Design review of the part built by this model. Coordinates are the model's own, in mm. A direction names the side the tool comes from. Coordinates: 2 decimals unless noted, no trailing zeros. Loops run counter-clockwise (first coordinate to the right, second up) from the corner with the lowest first, then second, coordinate; pieces in that order, holes last. Notation, with made-up numbers: M -11.75,-27 L 8.25,-27 A21 cw 8.25,-7 Z; hole C -22.75,57 d6. An arc over 180 degrees is marked long. Write item = value, one per line. Start each with the question number.
from build123d import *

# Parameters (mm, degrees)
SKETCH1_W                = 30
SKETCH1_H                = 80
BOSS_EXTRUDE1_DEPTH      = 5
SKETCH2_W                = 10
SKETCH2_H                = 10
BOSS_EXTRUDE2_DEPTH      = 30
CUT_EXTRUDE1_DEPTH       = 51.990195136
CUT_EXTRUDE1_DEPTH_BACK  = 51.990195136
SKETCH3_R                = 0.5
CUT_EXTRUDE2_DEPTH       = 46.276925691
CUT_EXTRUDE2_DEPTH_BACK  = 46.276925691
SKETCH4_W                = 25
SKETCH4_H                = 55
CUT_EXTRUDE3_DEPTH       = 83.006097334
CUT_EXTRUDE3_DEPTH_BACK  = 83.006097334
SKETCH5_W                = 26
SKETCH5_H                = 10
SKETCH6_W                = 10
SKETCH6_H                = 10
BOSS_EXTRUDE3_DEPTH      = 80
CUT_EXTRUDE4_DEPTH       = 83.006097334
CUT_EXTRUDE4_DEPTH_BACK  = 83.006097334
SKETCH7_R                = 1
CUT_EXTRUDE5_DEPTH       = 46.82575695
CUT_EXTRUDE5_DEPTH_BACK  = 46.82575695
SKETCH8_W                = 56
SKETCH8_H                = 10
SKETCH9_W                = 10
SKETCH9_H                = 10
CUT_EXTRUDE6_DEPTH       = 10
SKETCH10_W               = 10
SKETCH10_H               = 10
CUT_EXTRUDE7_DEPTH       = 10
SKETCH12_W               = 10
SKETCH12_H               = 2
BOSS_EXTRUDE5_DEPTH      = 10
CUT_EXTRUDE8_DEPTH       = 73.665328734
CUT_EXTRUDE8_DEPTH_BACK  = 73.665328734
SKETCH13_R               = 1
CUT_EXTRUDE11_DEPTH      = 46.276925691
CUT_EXTRUDE11_DEPTH_BACK = 46.276925691
SKETCH15_W               = 2
SKETCH15_H               = 2
SKETCH16_W               = 10
SKETCH16_H               = 10
BOSS_EXTRUDE6_DEPTH      = 30
SKETCH17_W               = 10
SKETCH17_H               = 10
CUT_EXTRUDE12_DEPTH      = 28
CUT_EXTRUDE13_DEPTH      = 48.053161424
CUT_EXTRUDE13_DEPTH_BACK = 48.053161424
SKETCH18_R               = 1
SKETCH20_W               = 10
SKETCH20_H               = 2
BOSS_EXTRUDE7_DEPTH      = 40


with BuildPart() as part:
    # Sketch1 → Boss-Extrude1 (new body)
    with BuildSketch(Plane(origin=(0, 0, 0), x_dir=(1, 0, 0), z_dir=(0, 1, 0))):
        Rectangle(SKETCH1_W, SKETCH1_H)
    extrude(amount=BOSS_EXTRUDE1_DEPTH)

    # Sketch2 → Boss-Extrude2 (add)
    with BuildSketch(Plane(origin=(15, 0, 0), x_dir=(0, 0, -1), z_dir=(1, 0, 0))):
        with Locations((-35, -5)):
            Rectangle(SKETCH2_W, SKETCH2_H)
        with Locations((35, -5)):
            Rectangle(SKETCH2_W, SKETCH2_H)
    extrude(amount=-BOSS_EXTRUDE2_DEPTH)

    # Sketch3 → Cut-Extrude1 (cut, two sides: drawn at the far end of the back side and taken through both)
    with BuildSketch(Plane(origin=(15, 0, 0), x_dir=(0, 0, -1), z_dir=(1, 0, 0)).offset(-CUT_EXTRUDE1_DEPTH_BACK)):
        with Locations((-35, -5)):
            Circle(SKETCH3_R)
        with Locations((35, -5)):
            Circle(SKETCH3_R)
    extrude(amount=CUT_EXTRUDE1_DEPTH + CUT_EXTRUDE1_DEPTH_BACK, mode=Mode.SUBTRACT)

    # Sketch4 → Cut-Extrude2 (cut, two sides: drawn at the far end of the back side and taken through both)
    with BuildSketch(Plane(origin=(0, 5, 0), x_dir=(1, 0, 0), z_dir=(0, 1, 0)).offset(-CUT_EXTRUDE2_DEPTH_BACK)):
        Rectangle(SKETCH4_W, SKETCH4_H)
    extrude(amount=CUT_EXTRUDE2_DEPTH + CUT_EXTRUDE2_DEPTH_BACK, mode=Mode.SUBTRACT)

    # Sketch5 → Cut-Extrude3 (cut, two sides: drawn at the far end of the back side and taken through both)
    with BuildSketch(Plane(origin=(0, 0, -40), x_dir=(-1, 0, 0), z_dir=(0, 0, -1)).offset(-CUT_EXTRUDE3_DEPTH_BACK)):
        with Locations((0, -5)):
            Rectangle(SKETCH5_W, SKETCH5_H)
    extrude(amount=CUT_EXTRUDE3_DEPTH + CUT_EXTRUDE3_DEPTH_BACK, mode=Mode.SUBTRACT)

    # Sketch6 → Boss-Extrude3 (add)
    with BuildSketch(Plane(origin=(0, 0, -40), x_dir=(-1, 0, 0), z_dir=(0, 0, -1))):
        with Locations((0, -5)):
            Rectangle(SKETCH6_W, SKETCH6_H)
    extrude(amount=-BOSS_EXTRUDE3_DEPTH)

    # Sketch7 → Cut-Extrude4 (cut, two sides: drawn at the far end of the back side and taken through both)
    with BuildSketch(Plane(origin=(0, 0, -40), x_dir=(-1, 0, 0), z_dir=(0, 0, -1)).offset(-CUT_EXTRUDE4_DEPTH_BACK)):
        with Locations((0, -5)):
            Circle(SKETCH7_R)
    extrude(amount=CUT_EXTRUDE4_DEPTH + CUT_EXTRUDE4_DEPTH_BACK, mode=Mode.SUBTRACT)

    # Sketch8 → Cut-Extrude5 (cut, two sides: drawn at the far end of the back side and taken through both)
    with BuildSketch(Plane(origin=(5, 0, 0), x_dir=(0, 0, -1), z_dir=(1, 0, 0)).offset(-CUT_EXTRUDE5_DEPTH_BACK)):
        with Locations((0, -5)):
            Rectangle(SKETCH8_W, SKETCH8_H)
    extrude(amount=CUT_EXTRUDE5_DEPTH + CUT_EXTRUDE5_DEPTH_BACK, mode=Mode.SUBTRACT)

    # Sketch9 → Cut-Extrude6 (cut)
    with BuildSketch(Plane.XY.offset(40)):
        with Locations((0, -5)):
            Rectangle(SKETCH9_W, SKETCH9_H)
    extrude(amount=-CUT_EXTRUDE6_DEPTH, mode=Mode.SUBTRACT)

    # Sketch10 → Cut-Extrude7 (cut)
    with BuildSketch(Plane(origin=(0, 0, -40), x_dir=(-1, 0, 0), z_dir=(0, 0, -1))):
        with Locations((0, -5)):
            Rectangle(SKETCH10_W, SKETCH10_H)
    extrude(amount=-CUT_EXTRUDE7_DEPTH, mode=Mode.SUBTRACT)

    # Sketch12 → Boss-Extrude5 (add)
    with BuildSketch(Plane(origin=(0, 5, 0), x_dir=(1, 0, 0), z_dir=(0, 1, 0))):
        with Locations((0, -28.5)):
            Rectangle(SKETCH12_W, SKETCH12_H)
        with Locations((0, 28.5)):
            Rectangle(SKETCH12_W, SKETCH12_H)
    extrude(amount=BOSS_EXTRUDE5_DEPTH)

    # Sketch13 → Cut-Extrude8 (cut, two sides: drawn at the far end of the back side and taken through both)
    with BuildSketch(Plane.XY.offset(29.5).offset(-CUT_EXTRUDE8_DEPTH_BACK)):
        with Locations((0, 10)):
            Circle(SKETCH13_R)
    extrude(amount=CUT_EXTRUDE8_DEPTH + CUT_EXTRUDE8_DEPTH_BACK, mode=Mode.SUBTRACT)

    # Sketch15 → Cut-Extrude11 (cut, two sides: drawn at the far end of the back side and taken through both)
    with BuildSketch(Plane(origin=(0, 5, 0), x_dir=(1, 0, 0), z_dir=(0, 1, 0)).offset(-CUT_EXTRUDE11_DEPTH_BACK)):
        with Locations((0, 33.5)):
            Rectangle(SKETCH15_W, SKETCH15_H)
    extrude(amount=CUT_EXTRUDE11_DEPTH + CUT_EXTRUDE11_DEPTH_BACK, mode=Mode.SUBTRACT)

    # Sketch16 → Boss-Extrude6 (add)
    with BuildSketch(Plane(origin=(0, 0, -30), x_dir=(-1, 0, 0), z_dir=(0, 0, -1))):
        with Locations((0, -5)):
            Rectangle(SKETCH16_W, SKETCH16_H)
    extrude(amount=-BOSS_EXTRUDE6_DEPTH)

    # Sketch17 → Cut-Extrude12 (cut)
    with BuildSketch(Plane(origin=(0, 0, -30), x_dir=(-1, 0, 0), z_dir=(0, 0, -1))):
        with Locations((0, -5)):
            Rectangle(SKETCH17_W, SKETCH17_H)
    extrude(amount=-CUT_EXTRUDE12_DEPTH, mode=Mode.SUBTRACT)


with BuildPart() as cut_extrude12_piece_1:
    # of the separate pieces the step leaves, piece 1, a body of its own (cut_extrude12_pieces)
    add(part.part.solids().sort_by_distance((-13, -10, -40))[0])



with BuildPart() as cut_extrude12_piece_2:
    # of the separate pieces the step leaves, piece 2, a body of its own (cut_extrude12_pieces)
    add(part.part.solids().sort_by_distance((-5, 0, -2))[0])

    # Sketch18 → Cut-Extrude13 (cut, two sides: drawn at the far end of the back side and taken through both)
    with BuildSketch(Plane(origin=(0, 0, -2), x_dir=(-1, 0, 0), z_dir=(0, 0, -1)).offset(-CUT_EXTRUDE13_DEPTH_BACK)):
        with Locations((0, -5)):
            Circle(SKETCH18_R)
    extrude(amount=CUT_EXTRUDE13_DEPTH + CUT_EXTRUDE13_DEPTH_BACK, mode=Mode.SUBTRACT)


with BuildPart() as cut_extrude12_piece_1_1:
    add(cut_extrude12_piece_1.part)

    add(cut_extrude12_piece_2.part)  # Boss-Extrude7 merges Cut-Extrude12 piece 2
    # Sketch20 → Boss-Extrude7 (add)
    with BuildSketch(Plane(origin=(0, 0, -40), x_dir=(-1, 0, 0), z_dir=(0, 0, -1))):
        with Locations((0, 1)):
            Rectangle(SKETCH20_W, SKETCH20_H)
    extrude(amount=-BOSS_EXTRUDE7_DEPTH)


solid = cut_extrude12_piece_1_1.part
Q1. Add section C-C on z = -20. State the section outline as (x, y) points.
Q2. Add section B-B on y = -7. State the section outline as (x, z) points.
Q3. Add section A-A on x = -9.5. State the section outline as (y, z) points.
Q4. To check wall thickness, follow line 1 (Z direction, x = 14.05, y = -5); line 2 (Y direction, x = 0, z = 29.15); line 3 (Z direction, x = -2.25, y = 9). State the ranges of each line that lie inside material, in increasing order. Write a range as from..to.
Q5. Clearance check with flat-ended pins moving along their axes: P1, Ø2.5, axis at x = 0, y = -5, coming from the -Z side; P2, Ø1, axis at y = 7.5, z = 28.5, coming from the -X side; P3, Ø5, axis at x = 1, z = -16, coming from the +Y side; P4, Ø4, axis at y = -0.5, z = -19, coming from the +X side. State where each tip first meets the part, or that it passes through.
Q6. Add section D-D on y = 6. State the section outline as (x, z) points.
Q7. For faces 1 (the face through (14, -5, 30)), 2 (the face through (14, -5, -30)), 3 (the face through (0, 3, -32.5)), 4 (the face through (5, 0.4, -9.7)), list the 3-axis set-ups (+Z, -Z, +X, -X, +Y, -Y) from which the entire face can be reached by the end or side of a thin tool; tool diameter is ignored.
Q8. Mouldability with a two-part tool opening along X and no side actions: class faces 5 (the face through (-14, -10, -35)), 6 (the face through (-1, 3, -33)), 7 (the face through (5, 10, -28)) as released by +X, released by -X, zero draft, split by the parting line, or undercut.
Values follow:
q1.outline = M -15,0 L -12.5,0 L -12.5,5 L -15,5 Z; M -5,0 L 5,0 L 5,2 L -5,2 Z; M 12.5,0 L 15,0 L 15,5 L 12.5,5 Z
q2.outline = M -15,-40 L -13,-40 L -13,-30 L -15,-30 Z; M -15,30 L -13,30 L -13,40 L -15,40 Z; M -5,-2 L 5,-2 L 5,0 L -5,0 Z; M -5,28 L 5,28 L 5,30 L -5,30 Z; M 13,-40 L 15,-40 L 15,-30 L 13,-30 Z; M 13,30 L 15,30 L 15,40 L 13,40 Z
q3.outline = M 0,-40 L 5,-40 L 5,-27.5 L 0,-27.5 Z; M 0,27.5 L 5,27.5 L 5,40 L 0,40 Z
q4.line_1 = -40..-35.5, -34.5..-30, 30..34.5, 35.5..40
q4.line_2 = -10..-6, -4..9, 11..15
q4.line_3 = -29.5..-27.5, 27.5..29.5
q5.P1 = -2
q5.P2 = -5
q5.P3 = 2
q5.P4 = 15
q6.outline = M -5,-29.5 L 5,-29.5 L 5,-27.5 L -5,-27.5 Z; M -5,27.5 L 5,27.5 L 5,29.5 L -5,29.5 Z
q7.face_1 = +X, -Y
q7.face_2 = +X, -X, -Y
q7.face_3 = +Y
q7.face_4 = +Y, -Y
q8.face_5 = zero draft
q8.face_6 = undercut
q8.face_7 = released by +X
